Autodesk Inventor part; units mm, degrees
ref_plane "YZ Plane" through (0, 0, 0) normal (1, 0, 0) x (0, 1, 0)
ref_plane "XZ Plane" through (0, 0, 0) normal (0, 1, 0) x (-1, 0, 0)
ref_plane "XY Plane" through (0, 0, 0) normal (0, 0, 1) x (1, 0, 0)
sketch "Sketch1" plane through (0, 0, 0) normal (0, 0, 1) x (1, 0, 0)
  arc A0 (-5.1284, 30.1824) -> (-4.7861, 30.3893) centre (0.7317, 20.8733) ccw
  circle A1 centre (0.7317, 20.8733) radius 11
  circle A2 centre (-141.2963, -27.3767) radius 11
  line L0 (-141.2963, -27.3767) -> (0.7317, -27.3767)
  line L1 (0.7317, -27.3767) -> (0.7317, 20.8733)
  line L2 (-70.2823, -27.3767) -> (-70.2823, -8.3767)
  line L3 (-70.2823, -27.3767) -> (-70.2823, -46.3767)
  line L4 (-141.2963, -11.3767) -> (-149.2963, -11.3767)
  line L5 (-152.2963, -14.3767) -> (-152.2963, -27.3767)
  line L6 (-152.2963, -27.3767) -> (-152.2963, -40.3767)
  line L7 (-141.2963, -11.3767) -> (-138.2963, -11.3767)
  line L8 (-138.2963, -11.3767) -> (-138.2963, -8.3767)
  line L9 (-138.2963, -8.3767) -> (-70.2823, -8.3767)
  line L10 (-141.2963, -46.3767) -> (-70.2823, -46.3767)
  line L11 (-12.2683, 31.8733) -> (13.7317, 31.8733)
  line L12 (4.7317, -46.3767) -> (-70.2823, -46.3767)
  line L13 (-15.2683, -8.3767) -> (-70.2823, -8.3767)
  line L14 (-141.2963, -46.3767) -> (-141.2963, -43.3767)
  line L15 (-141.2963, -43.3767) -> (-149.2963, -43.3767)
  line L16 (-15.2683, 20.8733) -> (-15.2683, -8.3767)
  line L17 (-15.2683, 20.8733) -> (-15.2683, 28.8733)
  line L18 (-12.2683, 31.8733) -> (-12.2683, 31.8733)
  line L19 (16.7317, 20.8733) -> (16.7317, 28.8733)
  line L20 (16.7317, 20.8733) -> (16.7317, -34.3767)
  line L21 (16.7317, -34.3767) -> (4.7317, -46.3767)
  arc A3 (-149.2963, -11.3767) -> (-152.2963, -14.3767) centre (-149.2963, -14.3767) ccw
  arc A4 (-152.2963, -40.3767) -> (-149.2963, -43.3767) centre (-149.2963, -40.3767) ccw
  arc A5 (-12.2683, 31.8733) -> (-15.2683, 28.8733) centre (-12.2683, 28.8733) ccw
  arc A6 (16.7317, 28.8733) -> (13.7317, 31.8733) centre (13.7317, 28.8733) ccw
  point P0 (16.7317, -46.3767)
  dimension "d8" = 22
  dimension "d9" = 19
  dimension "d10" = 16
  dimension "d12" = 19
  dimension "d15" = 3
  dimension "d17" = 16
  dimension "d18" = 16
  dimension "d19" = 12
  dimension "d20" = 12
  dimension "d21" = 3
  dimension "d22" = 3
extrude "Extrusion1" add sketch "Sketch1" along normal mid plane 102
extrude "Extrusion4" add sketch "Sketch1" along normal mid plane 105.5 contours A1 A0 | A2
properties part number "Bicep"
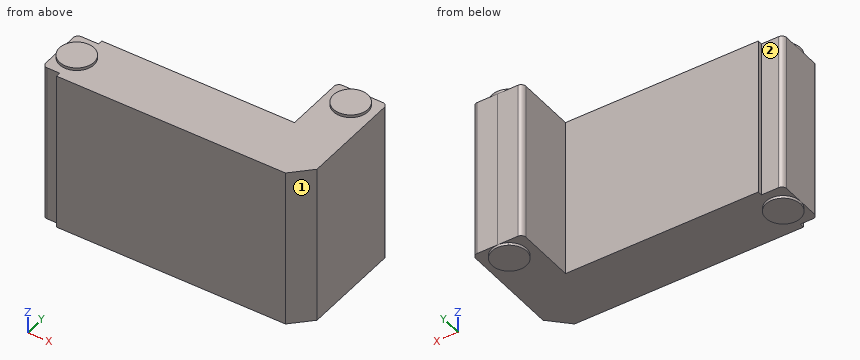
Input: part model. Units: mm. Frame: model coordinates. Face numbers are marked on the shaded views. A direction names the side the tool comes from. Coordinates: 2 decimals unless noted, no trailing zeros. Write each loop counter-clockwise with the first axis right and the second up, starting at its lowest first coordinate (ties: lowest second). Pieces come first, ordered by that corner, then holes.
1) Material intervals for line 1 along X through (y, z) = (3, 13.5); line 2 along Y through (x, z) = (-91.5, 23); line 3 along Z through (x, y) = (-47, -15.5), sorted ascending.
2) Set-up query: the marked faces 1 and 2. Return all of +Z, -Z, +X, -X, +Y, -Y with unobstructed straight access to the full face (end or side cutting, diameter ignored); none if empty.
3) Section A-A on z = -1. Output: boundary loops of the cut face in (x, y).
4) Section D-D on y = 20. Output: boundary loops of the cut face in (x, z), and give its area (3 significant figures).
5) Pin query (flat end, axial travel): pin 1 Ø0.9 at (y, z) = (-9, 4.5) entering from -X; pin 2 Ø6 at (y, z) = (10, -28.5) entering from -X; pin 3 Ø1 at (x, z) = (-69, -3.5) entering from +Y. Return the tip coordinate at first contact, or that it passes through.
6) Section C-C on x = -95.5. Output: boundary loops of the cut face in (y, z).
7) Section B-B on y = -31. Output: boundary loops of the cut face in (x, z).
Check result:
1. line 1: x = -15.27 to 16.73
1. line 2: y = -46.38 to -8.38
1. line 3: z = -51 to 51
2. face 1: +Z, -Z, +X, -Y
2. face 2: +Z, -Z, -X, +Y
3. outline: (-152.3, -40.38) arc R3 ccw to (-149.3, -43.38) - (-141.3, -43.38) - (-141.3, -46.38) - (4.73, -46.38) - (16.73, -34.38) - (16.73, 28.87) arc R3 ccw to (13.73, 31.87) - (0.79, 31.87) arc R11 ccw to (0.67, 31.87) - (-12.27, 31.87) arc R3 ccw to (-15.27, 28.87) - (-15.27, -8.38) - (-138.3, -8.38) - (-138.3, -11.38) - (-149.3, -11.38) arc R3 ccw to (-152.3, -14.38) - close
4. outline: (-15.27, -51) - (-10.23, -51) - (-10.23, -52.75) - (11.7, -52.75) - (11.7, -51) - (16.73, -51) - (16.73, 51) - (11.7, 51) - (11.7, 52.75) - (-10.23, 52.75) - (-10.23, 51) - (-15.27, 51) - close
4. area: 3,340 mm2
5. pin 1: stops at x = -138.3
5. pin 2: stops at x = -15.27
5. pin 3: stops at y = -8.38
6. outline: (-46.38, -51) - (-8.38, -51) - (-8.38, 51) - (-46.38, 51) - close
7. outline: (-152.3, -51) - (-151.68, -51) - (-151.68, -52.75) - (-130.91, -52.75) - (-130.91, -51) - (16.73, -51) - (16.73, 51) - (-130.91, 51) - (-130.91, 52.75) - (-151.68, 52.75) - (-151.68, 51) - (-152.3, 51) - close
